Read the model definition and answer for the solid it produces. Units are mm, in the model's axes. Give positions to 0.01 mm unless a question says otherwise; leave off trailing zeros. Loops run counter-clockwise (first coordinate to the right, second up) from the corner with the lowest first, then second, coordinate; pieces in that order, holes last.
(1) Determine the mould class of faces 1 (the face through (0.114, 1, -49)), 2 (the face through (-12, 1, -24.209)), 3 (the face through (-11.842, 0.986, -61.208)) for opening direction Z: pulls with the +Z half, pulls with the -Z half, needs draft (parallel to the pull), parting line crosses it, or undercut.
(2) Find section A-A, the plane y = 1.5. Write down the section's boundary in (x, z).
(3) Straight lines are drawn through the part: probe 1 along Z at (x, y) = (-11.75, 1.25); probe 2 along Z at (x, y) = (-2.5, 0.1); probe 3 along X at (y, z) = (1.65, -38). For each, find the intervals that lie inside material, in ascending order.
```python
from build123d import *

# Parameters (mm, degrees)
SKETCH_1_W          = 24
SKETCH_1_H          = 50
SKETCH_1_R          = 1
EXTRUDE_1_DEPTH     = 2
SKETCH_2_R          = 1
CUT_EXTRUDE_2_DEPTH = 2
CUT_EXTRUDE_3_DEPTH = 2


with BuildPart() as part:
    # 草图1 → 凸台-拉伸1 (new body)
    with BuildSketch(Plane(origin=(0, 0, 0), x_dir=(1, 0, 0), z_dir=(0, 1, 0))):
        with Locations((-11.885843957, 49.208625632)):
            Rectangle(SKETCH_1_W, SKETCH_1_H)
        with Locations(Location((-11.885843957, 60.208625632, 0), (0, 0, 270))):
            Circle(SKETCH_1_R, mode=Mode.SUBTRACT)
    extrude(amount=EXTRUDE_1_DEPTH)

    # 草图2 → 切除-拉伸2 (cut)
    with BuildSketch(Plane(origin=(0, 2, 0), x_dir=(1, 0, 0), z_dir=(0, 1, 0))):
        with Locations(Location((-11.885843957, 38.208625632, 0), (0, 0, 270))):
            Circle(SKETCH_2_R)
        with Locations(Location((-22.109843957, 72.412625632, 0), (0, 0, 270))):
            Circle(SKETCH_2_R)
        with Locations(Location((-1.655843957, 72.412625632, 0), (0, 0, 270))):
            Circle(SKETCH_2_R)
        with Locations(Location((-22.107843957, 25.986625632, 0), (0, 0, 270))):
            Circle(SKETCH_2_R)
        with Locations(Location((-1.655843957, 25.938625632, 0), (0, 0, 270))):
            Circle(SKETCH_2_R)
    extrude(amount=-CUT_EXTRUDE_2_DEPTH, mode=Mode.SUBTRACT)

    # 草图3 → 切除-拉伸3 (cut)
    with BuildSketch(Plane(origin=(0, 2, 0), x_dir=(1, 0, 0), z_dir=(0, 1, 0))):
        Polygon((-23.885843957, 74.208625632), (-23.535843957, 74.208625632), (-23.885843957, 73.858625632), align=None)
        Polygon((0.114156043, 74.208625632), (0.114156043, 73.858625632), (-0.235843957, 74.208625632), align=None)
        Polygon((0.114156043, 24.208625632), (-0.235843957, 24.208625632), (0.114156043, 24.558625632), align=None)
        Polygon((-23.885843957, 24.208625632), (-23.535843957, 24.208625632), (-23.885843957, 24.558625632), align=None)
    extrude(amount=-CUT_EXTRUDE_3_DEPTH, mode=Mode.SUBTRACT)


solid = part.part
```
Entries:
1. face 1: needs draft
1. face 2: pulls with the +Z half
1. face 3: undercut
2. outline: (-23.89, -73.86) - (-23.54, -74.21) - (-0.24, -74.21) - (0.11, -73.86) - (0.11, -24.56) - (-0.24, -24.21) - (-23.54, -24.21) - (-23.89, -24.56) - close; hole circle Ø2 at (-22.11, -72.41); hole circle Ø2 at (-22.11, -25.99); hole circle Ø2 at (-11.89, -60.21); hole circle Ø2 at (-11.89, -38.21); hole circle Ø2 at (-1.66, -72.41); hole circle Ø2 at (-1.66, -25.94)
3. probe 1: z = -74.21 to -61.2, -59.22 to -39.2, -37.22 to -24.21
3. probe 2: z = -74.21 to -72.95, -71.88 to -26.47, -25.4 to -24.21
3. probe 3: x = -23.89 to -12.86, -10.91 to 0.11
